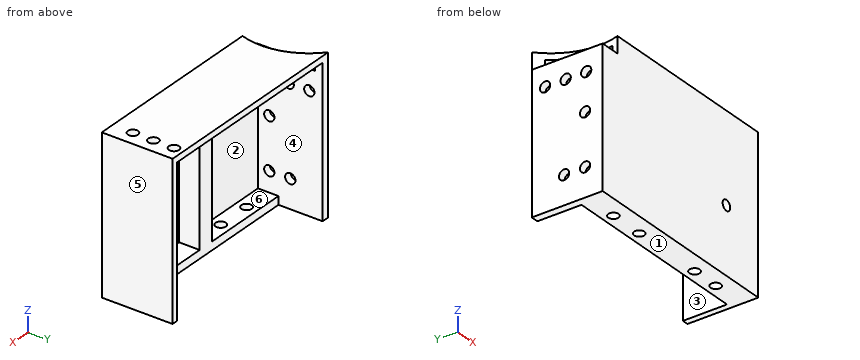
from build123d import *

# Parameters (mm, degrees)
CUBE_W                    = 150
CUBE_H                    = 150
BOSS_EXTRU_1_DEPTH        = 34.5
PAVE_W                    = 96
PAVE_H                    = 144
ENL_V_MAT_EXTRU_1_DEPTH   = 31.5
VIS1_R                    = 2.5
ENL_V_MAT_EXTRU_2_DEPTH   = 5
ENL_V_START               = -5
VIS2_R                    = 2.5
ENL_V_MAT_EXTRU_3_DEPTH   = 5
PAVE_PROCHE_MOTEUR_W      = 12.5
PAVE_PROCHE_MOTEUR_H      = 124
ENL_V_MAT_EXTRU_4_DEPTH   = 31.5
PAVE_ROUE_LIBRE_W         = 32.86
PAVE_ROUE_LIBRE_H         = 15.696676457
PAVE_ROUE_LIBRE_H_2       = 18.419496328
ENL_V_MAT_EXTRU_5_DEPTH   = 36
CABLES_W                  = 22.36
CABLES_H                  = 10
ENL_V_MAT_EXTRU_6_DEPTH   = 36
ROUE_EXT_R                = 32
ENL_V_MAT_EXTRU_7_DEPTH   = 8
ROUE_INTER_R              = 16.02
ENL_V_MAT_EXTRU_8_DEPTH   = 69
ENL_V_START_2             = -7.5
ROUE_EXT2_R               = 32
ENL_V_MAT_EXTRU_9_DEPTH   = 7.5
ENL_V_START_3             = -69
ROUE_INTER2_R             = 16.02
ENL_V_MAT_EXTRU_10_DEPTH  = 69
VIS_MOTEUR_POUR_SUPPORT_R = 2.5
ENL_V_MAT_EXTRU_11_DEPTH  = 10
BOSS_EXTRU_2_DEPTH        = 10
ESQUISSE2_R               = 2.5
ENL_V_MAT_EXTRU_12_DEPTH  = 10
ESQUISSE3_W               = 3.439870431
ESQUISSE3_H               = 124
BOSS_EXTRU_3_DEPTH        = 31
ESQUISSE5_W               = 3.439870431
ESQUISSE5_H               = 124
BOSS_EXTRU_4_DEPTH        = 0.5
ESQUISSE6_R               = 2.5
ENL_V_MAT_EXTRU_13_DEPTH  = 10
ESQUISSE7_R               = 2.5
ENL_V_MAT_EXTRU_14_DEPTH  = 10
ESQUISSE8_R               = 2.5
ENL_V_MAT_EXTRU_15_DEPTH  = 10
ENL_V_MAT_EXTRU_17_DEPTH  = 40


with BuildPart() as part:
    # Cube → Boss.-Extru.1 (new body)
    with BuildSketch(Plane(origin=(0, 0, 0), x_dir=(1, 0, 0), z_dir=(0, 1, 0))):
        with Locations((-34.210526316, -11.513157895)):
            Rectangle(CUBE_W, CUBE_H)
    extrude(amount=BOSS_EXTRU_1_DEPTH)

    # Pave → Enlèv. mat.-Extru.1 (cut)
    with BuildSketch(Plane(origin=(0, 34.5, 0), x_dir=(1, 0, 0), z_dir=(0, 1, 0))):
        with Locations((-10.210526316, -11.513157895)):
            Rectangle(PAVE_W, PAVE_H)
    extrude(amount=-ENL_V_MAT_EXTRU_1_DEPTH, mode=Mode.SUBTRACT)

    # Vis1 → Enlèv. mat.-Extru.2 (cut)
    with BuildSketch(Plane.XY.offset(86.513157895)):
        with Locations((33.789473684, 10)):
            Circle(VIS1_R)
        with Locations((33.789473684, 20)):
            Circle(VIS1_R)
        with Locations((33.789473684, 30)):
            Circle(VIS1_R)
    extrude(amount=-ENL_V_MAT_EXTRU_2_DEPTH, mode=Mode.SUBTRACT)

    # Vis2 → Enlèv. mat.-Extru.3 (cut)
    with BuildSketch(Plane(origin=(0, 0, -63.486842105), x_dir=(-1, 0, 0), z_dir=(0, 0, -1)).offset(ENL_V_START)):
        with Locations(Location((-33.789473684, 10, 0), (0, 0, 180))):
            Circle(VIS2_R)
        with Locations(Location((-33.789473684, 20, 0), (0, 0, 180))):
            Circle(VIS2_R)
        with Locations(Location((-33.789473684, 30, 0), (0, 0, 180))):
            Circle(VIS2_R)
    extrude(amount=ENL_V_MAT_EXTRU_3_DEPTH, mode=Mode.SUBTRACT)

    # Pave proche moteur → Enlèv. mat.-Extru.4 (cut)
    with BuildSketch(Plane(origin=(0, 34.5, 0), x_dir=(1, 0, 0), z_dir=(0, 1, 0))):
        with Locations((-67.460526316, -11.513157895)):
            Rectangle(PAVE_PROCHE_MOTEUR_W, PAVE_PROCHE_MOTEUR_H)
    extrude(amount=-ENL_V_MAT_EXTRU_4_DEPTH, mode=Mode.SUBTRACT)

    # Pave Roue libre → Enlèv. mat.-Extru.5 (cut)
    with BuildSketch(Plane(origin=(0, 34.5, 0), x_dir=(1, 0, 0), z_dir=(0, 1, 0))):
        with Locations((-87.980526316, 61.335180334)):
            Rectangle(PAVE_ROUE_LIBRE_W, PAVE_ROUE_LIBRE_H)
        with Locations((-87.980526316, -85.722906059)):
            Rectangle(PAVE_ROUE_LIBRE_W, PAVE_ROUE_LIBRE_H_2)
    extrude(amount=-ENL_V_MAT_EXTRU_5_DEPTH, mode=Mode.SUBTRACT)

    # Cables → Enlèv. mat.-Extru.6 (cut)
    with BuildSketch(Plane(origin=(0, 34.5, 0), x_dir=(1, 0, 0), z_dir=(0, 1, 0))):
        with Locations((-89.710526316, -0.513157895)):
            Rectangle(CABLES_W, CABLES_H)
        with Locations((-89.710526316, -22.513157895)):
            Rectangle(CABLES_W, CABLES_H)
    extrude(amount=-ENL_V_MAT_EXTRU_6_DEPTH, mode=Mode.SUBTRACT)

    # Roue ext → Enlèv. mat.-Extru.7 (cut)
    with BuildSketch(Plane.XY.offset(86.513157895)):
        with Locations((-82.5, 10)):
            Circle(ROUE_EXT_R)
    extrude(amount=-ENL_V_MAT_EXTRU_7_DEPTH, mode=Mode.SUBTRACT)

    # Roue inter → Enlèv. mat.-Extru.8 (cut)
    with BuildSketch(Plane.XY.offset(86.513157895)):
        with Locations((-82.5, 10)):
            Circle(ROUE_INTER_R)
    extrude(amount=-ENL_V_MAT_EXTRU_8_DEPTH, mode=Mode.SUBTRACT)

    # Roue ext2 → Enlèv. mat.-Extru.9 (cut)
    with BuildSketch(Plane(origin=(0, 0, -63.486842105), x_dir=(-1, 0, 0), z_dir=(0, 0, -1)).offset(ENL_V_START_2)):
        with Locations((82.5, 10)):
            Circle(ROUE_EXT2_R)
    extrude(amount=ENL_V_MAT_EXTRU_9_DEPTH, mode=Mode.SUBTRACT)

    # Roue inter2 → Enlèv. mat.-Extru.10 (cut)
    with BuildSketch(Plane(origin=(0, 0, -63.486842105), x_dir=(-1, 0, 0), z_dir=(0, 0, -1)).offset(ENL_V_START_3)):
        with Locations((82.5, 10)):
            Circle(ROUE_INTER2_R)
    extrude(amount=ENL_V_MAT_EXTRU_10_DEPTH, mode=Mode.SUBTRACT)

    # Vis Moteur pour support → Enlèv. mat.-Extru.11 (cut)
    with BuildSketch(Plane(origin=(-58.210526316, 0, 0), x_dir=(0, 0, -1), z_dir=(1, 0, 0))):
        with Locations((-68.513157895, 8)):
            Circle(VIS_MOTEUR_POUR_SUPPORT_R)
        with Locations((-68.513157895, 18)):
            Circle(VIS_MOTEUR_POUR_SUPPORT_R)
        with Locations((-68.513157895, 28)):
            Circle(VIS_MOTEUR_POUR_SUPPORT_R)
        with Locations((45.986842105, 8)):
            Circle(VIS_MOTEUR_POUR_SUPPORT_R)
        with Locations((45.986842105, 18)):
            Circle(VIS_MOTEUR_POUR_SUPPORT_R)
        with Locations((45.986842105, 28)):
            Circle(VIS_MOTEUR_POUR_SUPPORT_R)
    extrude(amount=-ENL_V_MAT_EXTRU_11_DEPTH, mode=Mode.SUBTRACT)

    # Esquisse1 → Boss.-Extru.2 (add)
    with BuildSketch(Plane(origin=(0, 3, 0), x_dir=(1, 0, 0), z_dir=(0, 1, 0))):
        Polygon((-58.210526316, -15.513157895), (-14.210526316, -15.513157895), (-14.210526316, -83.513157895), (-6.210526316, -83.513157895), (-6.210526316, -15.513157895), (37.789473684, -15.513157895), (37.789473684, -7.513157895), (-6.210526316, -7.513157895), (-6.210526316, 60.486842105), (-14.210526316, 60.486842105), (-14.210526316, -7.513157895), (-58.210526316, -7.513157895), align=None)
    extrude(amount=BOSS_EXTRU_2_DEPTH)

    # Esquisse2 → Enlèv. mat.-Extru.12 (cut)
    with BuildSketch(Plane.XY.offset(15.513157895)):
        with Locations((-43.942882256, 8)):
            Circle(ESQUISSE2_R)
        with Locations((-26.88958752, 8)):
            Circle(ESQUISSE2_R)
        with Locations((9.588466595, 8)):
            Circle(ESQUISSE2_R)
        with Locations((23.56238511, 8)):
            Circle(ESQUISSE2_R)
    extrude(amount=-ENL_V_MAT_EXTRU_12_DEPTH, mode=Mode.SUBTRACT)

    # Esquisse3 → Boss.-Extru.3 (add)
    with BuildSketch(Plane(origin=(0, 3, 0), x_dir=(1, 0, 0), z_dir=(0, 1, 0))):
        with Locations((-62.930461532, -11.513157895)):
            Rectangle(ESQUISSE3_W, ESQUISSE3_H)
    extrude(amount=BOSS_EXTRU_3_DEPTH)

    # Esquisse5 → Boss.-Extru.4 (add)
    with BuildSketch(Plane(origin=(0, 34, 0), x_dir=(1, 0, 0), z_dir=(0, 1, 0))):
        with Locations((-62.930461532, -11.513157895)):
            Rectangle(ESQUISSE5_W, ESQUISSE5_H)
    extrude(amount=BOSS_EXTRU_4_DEPTH)

    # Esquisse6 → Enlèv. mat.-Extru.13 (cut)
    with BuildSketch(Plane(origin=(-58.210526316, 0, 0), x_dir=(0, 0, -1), z_dir=(1, 0, 0))):
        with Locations((-68.513157895, 28)):
            Circle(ESQUISSE6_R)
        with Locations((-68.513157895, 18)):
            Circle(ESQUISSE6_R)
        with Locations((-68.513157895, 8)):
            Circle(ESQUISSE6_R)
        with Locations((45.986842105, 28)):
            Circle(ESQUISSE6_R)
        with Locations((45.986842105, 18)):
            Circle(ESQUISSE6_R)
        with Locations((45.986842105, 8)):
            Circle(ESQUISSE6_R)
    extrude(amount=-ENL_V_MAT_EXTRU_13_DEPTH, mode=Mode.SUBTRACT)

    # Esquisse7 → Enlèv. mat.-Extru.14 (cut)
    with BuildSketch(Plane(origin=(-58.210526316, 0, 0), x_dir=(0, 0, -1), z_dir=(1, 0, 0))):
        with Locations((0, 8.527871685)):
            Circle(ESQUISSE7_R)
        with Locations((0, 18.750861141)):
            Circle(ESQUISSE7_R)
        with Locations((-25.400224022, 8.527871685)):
            Circle(ESQUISSE7_R)
        with Locations((-25.400224022, 18.750861141)):
            Circle(ESQUISSE7_R)
        with Locations((-50.386538843, 8.527871685)):
            Circle(ESQUISSE7_R)
        with Locations((23.629525814, 8.527871685)):
            Circle(ESQUISSE7_R)
    extrude(amount=-ENL_V_MAT_EXTRU_14_DEPTH, mode=Mode.SUBTRACT)

    # Esquisse8 → Enlèv. mat.-Extru.15 (cut)
    with BuildSketch(Plane(origin=(0, 3, 0), x_dir=(1, 0, 0), z_dir=(0, 1, 0))):
        with Locations(Location((19.789473684, -43.513157895, 0), (0, 0, 270))):
            Circle(ESQUISSE8_R)
        with Locations(Location((19.789473684, 20.486842105, 0), (0, 0, 270))):
            Circle(ESQUISSE8_R)
    extrude(amount=-ENL_V_MAT_EXTRU_15_DEPTH, mode=Mode.SUBTRACT)

    # Esquisse9 → Enlèv. mat.-Extru.17 (cut)
    with BuildSketch(Plane(origin=(0, 34.5, 0), x_dir=(1, 0, 0), z_dir=(0, 1, 0))):
        Polygon((-61.91481115, -86.513157895), (-109.210526316, -86.513157895), (-109.210526316, 63.486842105), (-61.91481115, 63.486842105), (40.789473684, 63.486842105), (40.789473684, -11.513157895), (-61.91481115, -11.513157895), align=None)
    extrude(amount=-ENL_V_MAT_EXTRU_17_DEPTH, mode=Mode.SUBTRACT)


solid = part.part
The model under review builds one solid part; all positions refer to its coordinate system, in mm. Face numbers are marked on the shaded views. A direction names the side the tool comes from. Give positions to 0.01 mm unless a question says otherwise; leave off trailing zeros. Loops run counter-clockwise (first coordinate to the right, second up) from the corner with the lowest first, then second, coordinate; pieces in that order, holes last. Notation, with made-up numbers: (52.25, 62.5) -> (99.25, 62.5) arc R16 ccw to (99.25, 70.5) -> close; hole circle Ø11 at (-38.5, -5.5). An arc over 180 degrees is marked (long way). Put each result on its own line as item: value. Start each with the question number.
1. We need section B-B on z = 37. State the section outline as (x, y) points.
2. For the marked faces 5 and 6, list the 3-axis set-ups (+Z, -Z, +X, -X, +Y, -Y) from which the entire face can be reached by the end or side of a thin tool; tool diameter is ignored.
3. Wall thickness on probe 1 along X at (y, z) = (11.5, 28.5); probe 2 along Z at (x, y) = (17.5, 12.5); probe 3 along X at (y, z) = (15, 19.5): over which ranges is each line inside the solid? List them lowest first.
4. We need section A-A on x = -22.5. State the section outline as (y, z) points.
5. Mouldability with a two-part tool opening along Z and no side actions: class the marked faces 1, 2, 3 and 4 as released by +Z, released by -Z, zero draft, split by the parting line, or undercut.
6. Clearance check with flat-ended pins moving along their axes: P1, Ø13, axis at x = -27, z = 57, coming from the +Y side; P2, Ø11.5, axis at x = -57, y = 12.5, coming from the +Z side. State where each tip first meets the part, or that it passes through.
Determined:
1. outline: (-61.91, 0) -> (40.79, 0) -> (40.79, 34.5) -> (37.79, 34.5) -> (37.79, 3) -> (-6.21, 3) -> (-6.21, 13) -> (-14.21, 13) -> (-14.21, 3) -> (-58.21, 3) -> (-58.21, 34.5) -> (-61.91, 34.5) -> close
2. face 5: +Z, -Z, +X, +Y, -Y
2. face 6: +Y
3. probe 1: -61.91 to -58.21, -14.21 to -6.21, 37.79 to 40.79
3. probe 2: 11.51 to 15.51, 83.51 to 86.51
3. probe 3: -61.91 to -58.21, 37.79 to 40.79
4. outline: (0, 11.51) -> (13, 11.51) -> (13, 15.51) -> (3, 15.51) -> (3, 83.51) -> (34.5, 83.51) -> (34.5, 86.51) -> (0, 86.51) -> close
5. face 1: released by -Z
5. face 2: undercut
5. face 3: undercut
5. face 4: zero draft
6. P1: y = 3
6. P2: z = 78.51
